For this review, use the dimensioned drawing (mm, ordinates from the lowest corner) and the shaded views. A direction names the side the tool comes from. Round coordinates to 2 decimals unless told otherwise and drop trailing zeros. Order: outer loops, then holes, each group sorted by start corner. A loop starts at its lowest first (then second) coordinate and runs counter-clockwise, first axis right, second up. Notation, with made-up numbers: (17.5, 38) -> (71.5, 38) arc R28 ccw to (71.5, 57) -> close; hole circle Ø1 at (19, -40). An arc over 180 degrees is marked (long way). Use a Markdown table: item, result. Add a question column.
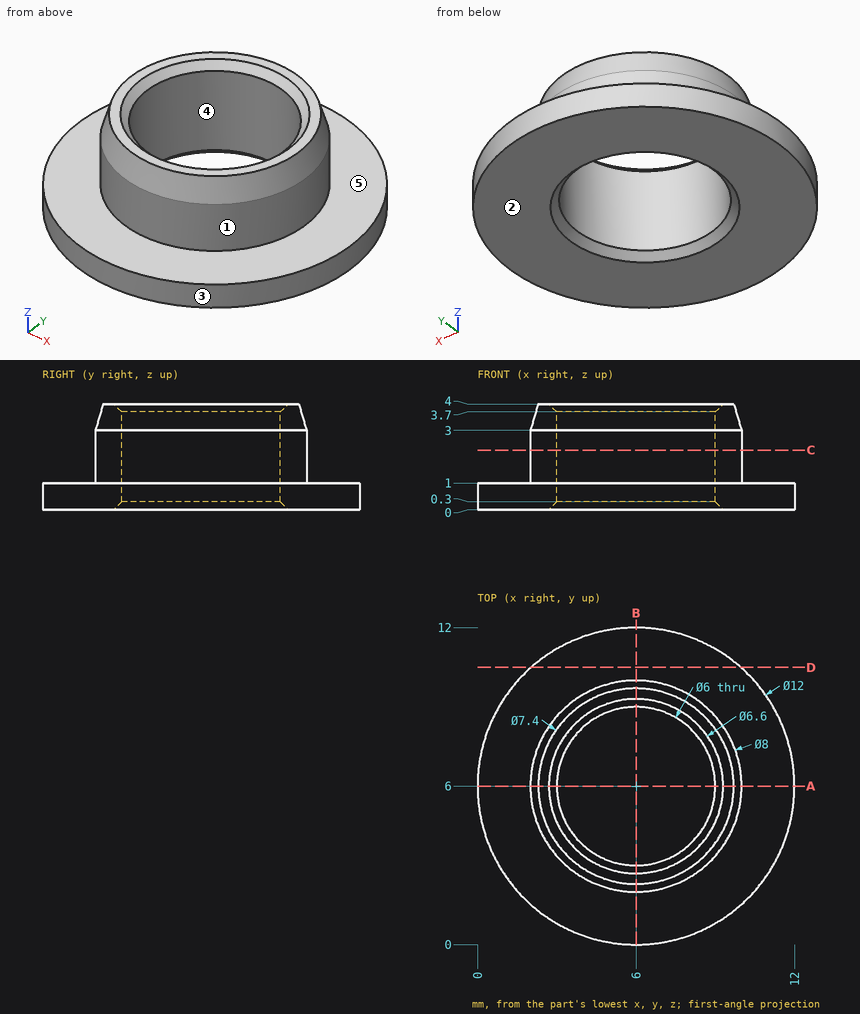
Q1. Machinability: for the marked faces 1 and 2, which of the approach directions +Z, -Z, +X, -X, +Y, -Y give a long, thin tool a straight path to every point of the face, cutting with its end or side? Answer none if there is none.
Q2. Mouldability with a two-part tool opening along X and no side actions: class the marked faces 3, 4 and 5 as pulls with the +X half, pulls with the -X half, needs draft (parallel to the pull), parting line crosses it, or undercut.
Q3. Add section A-A (y = 6). Write out the cut boundary in (x, z), then the cut area to 3 significant figures.
Q4. Insertion check: pin 1 (2 mm diameter, centred on y = 2.5, z = 3, fed in from -X). The pin has a flat end and moves straight along its axis. Give the tip position at first contact, or say it passes through.
Q5. Add section D-D (y = 10.5). Write out the cut boundary in (x, z), then the cut area to 3 significant figures.
Q6. Add section C-C (z = 2.25). Write out the cut boundary in (x, y).
Q7. Wall thickness on line 1 (Y direction, x = 6, z = 2.5); line 2 (Z direction, x = 2.5, y = 2.5); line 3 (X direction, y = 8, z = 3.85): over which ranges is each line inside the solid? List them lowest first. Write a range as [from, to].
Report:
| question | item | result |
|---|---|---|
| 1 | face 1 | +Z |
| 1 | face 2 | -Z, +X, -X, +Y, -Y |
| 2 | face 3 | parting line crosses it |
| 2 | face 4 | undercut |
| 2 | face 5 | needs draft |
| 3 | outline | (0, 0) -> (2.7, 0) -> (3, 0.3) -> (3, 3.7) -> (2.7, 4) -> (2.3, 4) -> (2, 3) -> (2, 1) -> (0, 1) -> close; (9, 0.3) -> (9.3, 0) -> (12, 0) -> (12, 1) -> (10, 1) -> (10, 3) -> (9.7, 4) -> (9.3, 4) -> (9, 3.7) -> close |
| 3 | area | 11.5 mm² |
| 4 | pin 1 | stops at x = 2.88 |
| 5 | outline | (2.03, 0) -> (9.97, 0) -> (9.97, 1) -> (2.03, 1) -> close |
| 5 | area | 7.94 mm² |
| 6 | outline | circle Ø8 at (6, 6); hole circle Ø6 at (6, 6) |
| 7 | line 1 | y = [2, 3], [9, 10] |
| 7 | line 2 | z = [0, 1] |
| 7 | line 3 | x = [2.83, 3.57], [8.43, 9.17] |
